```python
from build123d import *

# Parameters (mm, degrees)
BOSS_EXTRUDE2_DEPTH = 20
SKETCH4_R           = 10.1
CUT_EXTRUDE1_DEPTH  = 20
SKETCH5_R           = 10.1
CUT_EXTRUDE2_DEPTH  = 20
FILLET1_R           = 8
SCALE1_SCALE        = 0.5


with BuildPart() as part:
    # Sketch3 → Boss-Extrude2 (new body)
    with BuildSketch(Plane(origin=(0, 0, 0), x_dir=(0, 0, -1), z_dir=(1, 0, 0))):
        with BuildLine():
            Line((-17.320508076, -10), (-72.679491924, -10))
            ThreePointArc((-72.679491924, -10), (-110, 0), (-72.679491924, 10))
            Line((-72.679491924, 10), (-17.320508076, 10))
            ThreePointArc((-17.320508076, 10), (20, 0), (-17.320508076, -10))
        make_face()
    extrude(amount=BOSS_EXTRUDE2_DEPTH)

    # Sketch4 → Cut-Extrude1 (cut)
    with BuildSketch(Plane(origin=(0, 0, 0), x_dir=(0, 0, -1), z_dir=(1, 0, 0))):
        with Locations((-90, 0)):
            Circle(SKETCH4_R)
    extrude(amount=CUT_EXTRUDE1_DEPTH, mode=Mode.SUBTRACT)

    # Sketch5 → Cut-Extrude2 (cut)
    with BuildSketch(Plane(origin=(0, 0, 0), x_dir=(0, 0, -1), z_dir=(1, 0, 0))):
        Circle(SKETCH5_R)
    extrude(amount=CUT_EXTRUDE2_DEPTH, mode=Mode.SUBTRACT)

    # Fillet1
    fillet1_edges = [part.edges().sort_by_distance(p)[0] for p in [
        (20, 0, 110),
        (20, -10, 45),
        (20, 0, -20),
        (0, -10, 45),
        (0, 0, 110),
        (0, 10, 45),
        (0, 0, -20),
        (10, -10, 17.320508076),
        (10, -10, 72.679491924),
        (10, 10, 72.679491924),
        (10, 10, 17.320508076),
        (20, 10, 45),
    ]]
    fillet(fillet1_edges, radius=FILLET1_R)


with BuildPart() as part_1:
    # Scale1: scaled about (0, 0, 0)
    add(part.part.scale(SCALE1_SCALE))


solid = part_1.part
```
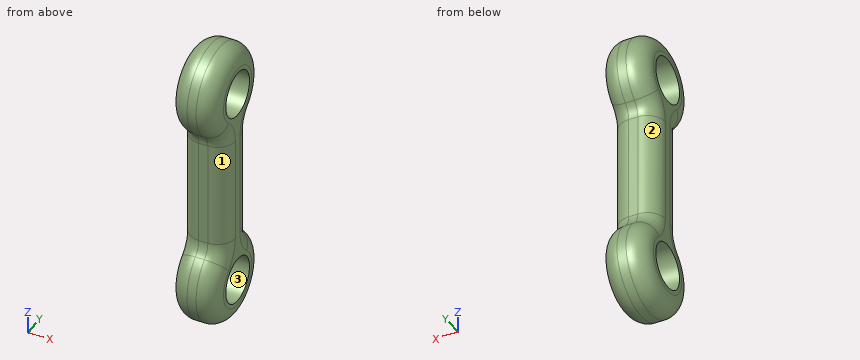
Could you check a few things on this model? Use its own coordinates, in mm. Face numbers are marked on the shaded views. A direction names the side the tool comes from. Coordinates: 2 decimals unless noted, no trailing zeros. Write each loop counter-clockwise with the first axis right and the second up, starting at its lowest first coordinate (ties: lowest second). Pieces come first, ordered by that corner, then holes. Notation, with made-up numbers: (-20.5, 1.5) -> (-11.5, 1.5) arc R33 cw to (-11.5, 37.5) -> close; hole circle Ø2 at (85, 41.5). An arc over 180 degrees is marked (long way). Return JSON: item names as keys, results as strings.
(1) I'm going to push flat-ended pins straight in: pin 1 (8 mm diameter, centred on y = 0, z = 0, fed in from +X); pin 2 (1 mm diameter, centred on x = 6, z = 29.5, fed in from +Y); pin 3 (4 mm diameter, centred on x = 8.5, z = 12, fed in from -Y); pin 4 (2 mm diameter, centred on x = 6.5, y = 3.5, fed in from -Z). Where does each tip first touch, or does it pass through?
Numbers:
{"pin 1": "passes through", "pin 2": "stops at y = 5", "pin 3": "stops at y = -4.97", "pin 4": "stops at z = -9.67"}
(2) Imagine slicing it at A-A, the plane y = 0. Please give me the cut outline in (x, z).
Numbers:
{"outline": "(0, -6) arc R4 ccw to (4, -10) -> (6, -10) arc R4 ccw to (10, -6) -> (10, -5.05) -> (0, -5.05) -> close; (0, 5.05) -> (10, 5.05) -> (10, 39.95) -> (0, 39.95) -> close; (0, 50.05) -> (10, 50.05) -> (10, 51) arc R4 ccw to (6, 55) -> (4, 55) arc R4 ccw to (0, 51) -> close"}
(3) Imagine slicing it at B-B, the plane z = 17. Please give me the cut outline in (x, y).
Numbers:
{"outline": "(0, -1) arc R4 ccw to (4, -5) -> (6, -5) arc R4 ccw to (10, -1) -> (10, 1) arc R4 ccw to (6, 5) -> (4, 5) arc R4 ccw to (0, 1) -> close"}
(4) I need wall thicknesses on L1, parallel to Y at x = 4, z = 0; L2, parallel to Z at x = 6, y = -2.75; L3, parallel to Z at x = 1.75, y = 4.25. Which ranges of each line are inside material? Lowest first, please.
Numbers:
{"L1": "y = -10 to -5.05, 5.05 to 10", "L2": "z = -9.61 to -4.24, 4.24 to 40.76, 49.24 to 54.61", "L3": "z = -8.28 to -2.73, 2.73 to 42.27, 47.73 to 53.28"}
(5) Which directions (+Z, -Z, +X, -X, +Y, -Y) give clear straight access to the entire face, cutting with the end or side of a thin tool? Please do the marked faces 1, 2 and 3.
Numbers:
{"face 1": "+X, -Y", "face 2": "-X, +Y", "face 3": "+X, -X"}
(6) Imagine slicing it at C-C, the plane y = 3. Count the separate pieces of the cut face and the enclosed holes in it, then the cut area to 3 significant figures.
Numbers:
{"separate pieces": "3", "enclosed holes": "0", "area": "433 mm2"}
